Here's how the part is built. I have some questions about the finished solid (model axes, mm). Coordinates: 2 decimals unless noted, no trailing zeros. Write each loop counter-clockwise with the first axis right and the second up, starting at its lowest first coordinate (ties: lowest second). Pieces come first, ordered by that corner, then holes. Notation, with made-up numbers: (-20.5, 36) -> (8.5, 36) arc R32 ccw to (8.5, 70) -> close; hole circle Ø11 at (38.25, -29.75). An arc over 180 degrees is marked (long way). Put each result on its own line as item: value.
```python
from build123d import *

# Parameters (mm, degrees)
SKETCH1_W               = 121
SKETCH1_H               = 60
SKETCH1_R               = 5
SKETCH1_R_2             = 2.83
BOSS_EXTRUDE1_DEPTH     = 4
SKETCH2_W               = 4
SKETCH2_H               = 60
BOSS_EXTRUDE2_DEPTH     = 4
CUT_EXTRUDE1_DEPTH      = 87.469647854
CUT_EXTRUDE1_DEPTH_BACK = 87.469647854
SKETCH3_R               = 1.75
SKETCH3_W               = 3.4
SKETCH3_H               = 8.7


with BuildPart() as part:
    # Sketch1 → Boss-Extrude1 (new body)
    with BuildSketch(Plane.XY):
        with Locations((-20.5, 0)):
            Rectangle(SKETCH1_W, SKETCH1_H)
        with Locations((-48, 0)):
            Circle(SKETCH1_R, mode=Mode.SUBTRACT)
        with Locations((23, -24)):
            Circle(SKETCH1_R_2, mode=Mode.SUBTRACT)
    extrude(amount=BOSS_EXTRUDE1_DEPTH)

    # Sketch2 → Boss-Extrude2 (add)
    with BuildSketch(Plane.XY):
        with Locations((42, 0)):
            Rectangle(SKETCH2_W, SKETCH2_H)
    extrude(amount=BOSS_EXTRUDE2_DEPTH)

    # Sketch3 → Cut-Extrude1 (cut, two sides: drawn at the far end of the back side and taken through both)
    with BuildSketch(Plane.XY.offset(-CUT_EXTRUDE1_DEPTH_BACK)):
        with Locations((-7, 0)):
            Circle(SKETCH3_R)
        with Locations((38.3, 21.65)):
            Rectangle(SKETCH3_W, SKETCH3_H)
        with Locations((38.3, -21.65)):
            Rectangle(SKETCH3_W, SKETCH3_H)
    extrude(amount=CUT_EXTRUDE1_DEPTH + CUT_EXTRUDE1_DEPTH_BACK, mode=Mode.SUBTRACT)


solid = part.part
```
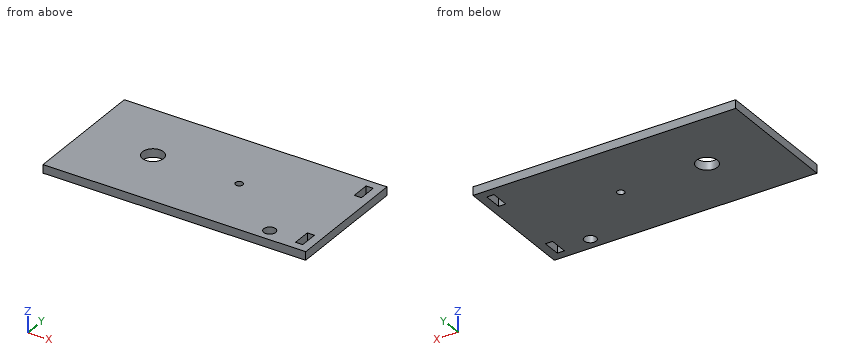
Item 1: Imagine slicing it at A-A on x = 23. Write out the boundary of the cut face in (y, z), then the cut area to 3 significant figures.
Output:
outline: (-30, 0) -> (-26.83, 0) -> (-26.83, 4) -> (-30, 4) -> close; (-21.17, 0) -> (30, 0) -> (30, 4) -> (-21.17, 4) -> close
area: 217 mm²
Item 2: Imagine slicing it at C-C on y = 0. Write out the boundary of the cut face in (x, z).
Output:
outline: (-81, 0) -> (-53, 0) -> (-53, 4) -> (-81, 4) -> close; (-43, 0) -> (-8.75, 0) -> (-8.75, 4) -> (-43, 4) -> close; (-5.25, 0) -> (44, 0) -> (44, 4) -> (-5.25, 4) -> close
Item 3: Imagine slicing it at D-D on z = 1.4. Write out the boundary of the cut face in (x, y).
Output:
outline: (-81, -30) -> (44, -30) -> (44, 30) -> (-81, 30) -> close; hole circle Ø10 at (-48, 0); hole circle Ø3.5 at (-7, 0); hole circle Ø5.66 at (23, -24); hole (36.6, -26) -> (40, -26) -> (40, -17.3) -> (36.6, -17.3) -> close; hole (36.6, 17.3) -> (40, 17.3) -> (40, 26) -> (36.6, 26) -> close
Item 4: Please list where these lines run through material, in increasing order: line 1 along Y through (x, z) = (38, 2.2); line 2 along Y through (x, z) = (-48, 1.65); line 3 along X through (y, z) = (24, 3.6). Write a range as from..to.
Output:
line 1: y = -30..-26, -17.3..17.3, 26..30
line 2: y = -30..-5, 5..30
line 3: x = -81..36.6, 40..44
Item 5: Imagine slicing it at B-B on y = -18.5. Write out the boundary of the cut face in (x, z).
Output:
outline: (-81, 0) -> (36.6, 0) -> (36.6, 4) -> (-81, 4) -> close; (40, 0) -> (44, 0) -> (44, 4) -> (40, 4) -> close
Item 6: For P1, Ø4, axis at x = -7, y = 0, coming from the -Z side, with a flat end and sliding along its axis, tell me the tip position at first contact or that it passes through.
Output:
P1: stops at z = 0
